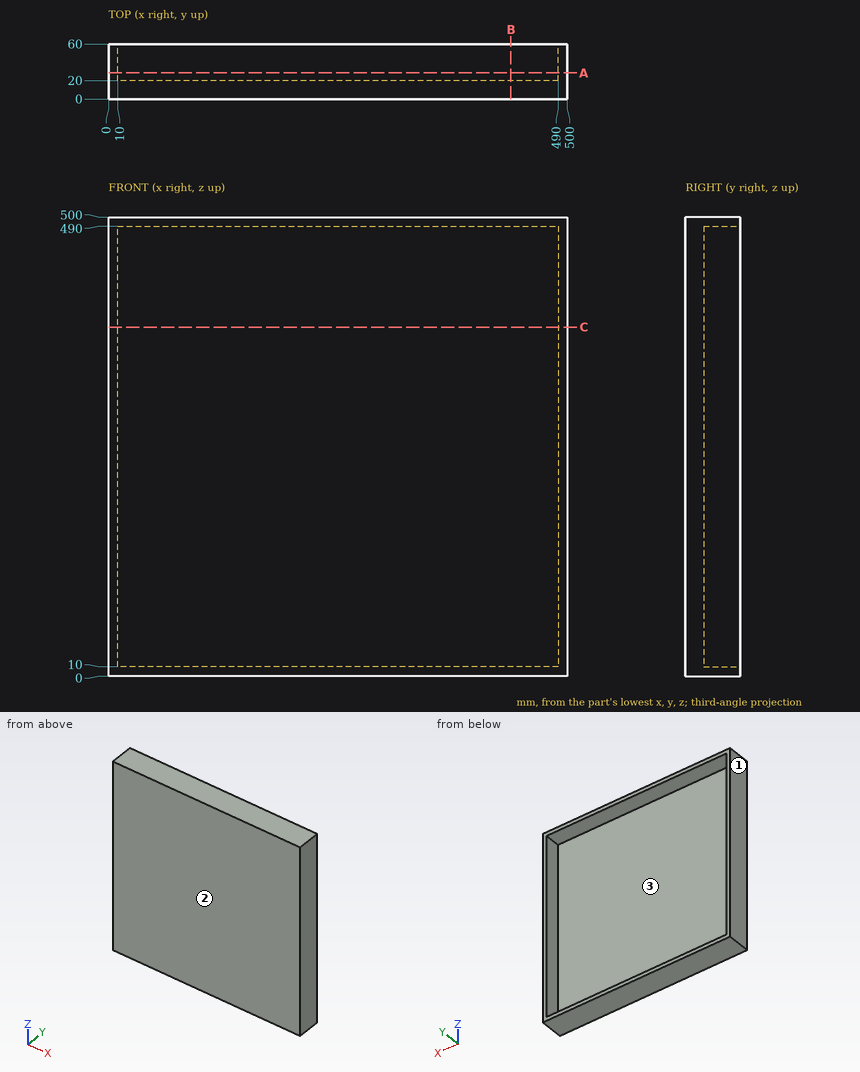
The drawing under review shows one solid part. Ordinate dimensions are in mm from its lowest x, y, z. Give positions to 0.01 mm unless a question says otherwise; leave off trailing zeros. Loops run counter-clockwise (first coordinate to the right, second up) from the corner with the lowest first, then second, coordinate; pieces in that order, holes last. Notation, with made-up numbers: M 8,35 L 25,35 A20 cw 25,57 Z; hole C 59.5,64.25 d4. An arc over 180 degrees is marked long. One line per item, written item: value. Start each with the question number.
Q1. Add section B-B (x = 438.5). Give the boundary of the cut face in (y, z).
Q2. Add section A-A (y = 28.5). Give the boundary of the cut face in (x, z).
Q3. Draft analysis for pull direction X (two halves, no side actions). For the marked faces 1, 2 and 3, state which applies: released by +X, released by -X, zero draft, split by the parting line, or undercut.
Q4. For L1, parallel to Z at x = 374.5, y = 27; L2, parallel to Y at x = 458, z = 197, list the stretches that pass through material, from the lowest coordinate up.
Q5. Add section C-C (z = 380). Give the boundary of the cut face in (x, y).
Reply:
1. outline: M 0,0 L 60,0 L 60,10 L 20,10 L 20,490 L 60,490 L 60,500 L 0,500 Z
2. outline: M 0,0 L 500,0 L 500,500 L 0,500 Z; hole M 10,10 L 490,10 L 490,490 L 10,490 Z
3. face 1: released by -X
3. face 2: zero draft
3. face 3: undercut
4. L1: 0 to 10, 490 to 500
4. L2: 0 to 20
5. outline: M 0,0 L 500,0 L 500,60 L 490,60 L 490,20 L 10,20 L 10,60 L 0,60 Z
